Here's the drawing with two shaded views (mm, measured from the low corner). I have some questions. Coordinates: 2 decimals unless noted, no trailing zeros. Loops run counter-clockwise (first coordinate to the right, second up) from the corner with the lowest first, then second, coordinate; pieces in that order, holes last. Notation, with made-up numbers: (-37, 66) -> (-22, 66) arc R27 ccw to (-22, 93) -> close; hole circle Ø1 at (11, 86.5). An arc over 180 degrees is marked (long way). Answer as a JSON object with one key per item and string values. Group by question number.
1) I want a section at D-D (y = 41). Write out the boundary of the cut face in (x, z), then the cut area to 3 significant figures.
2) I want a section at A-A (y = 25.5). Write out the boundary of the cut face in (x, z) (3 decimals).
3) I want a section at C-C (x = 0.7). Write out the boundary of the cut face in (y, z), then the cut area to 4 significant figures.
4) I need wall thicknesses on probe 1 along Z at (x, y) = (0.8, 32.5); probe 2 along Y at (x, z) = (4.6, 14). Which ranges of each line are inside material? Lowest first, please. Write a range as [from, to].
5) I'm going to push flat-ended pins straight in: pin 1 (3 mm diameter, centred on x = 4, z = 25.5, fed in from -Y); pin 2 (8 mm diameter, centred on y = 29, z = 23.5, fed in from -X); pin 3 (2 mm diameter, centred on x = 1, y = 32.5, fed in from +Z); pin 4 (0.8 mm diameter, centred on x = 1, y = 25, fed in from -Z). Where does each tip first touch, or does it pass through?
6) I want a section at B-B (z = 26). Write out the boundary of the cut face in (x, y).
7) If we mould it in two halves opening along Z, with no side actions, what happens to the marked faces 1 and 2? For each: +Z half, -Z half, draft (parallel to the pull), parting line (faces both ways), or undercut.
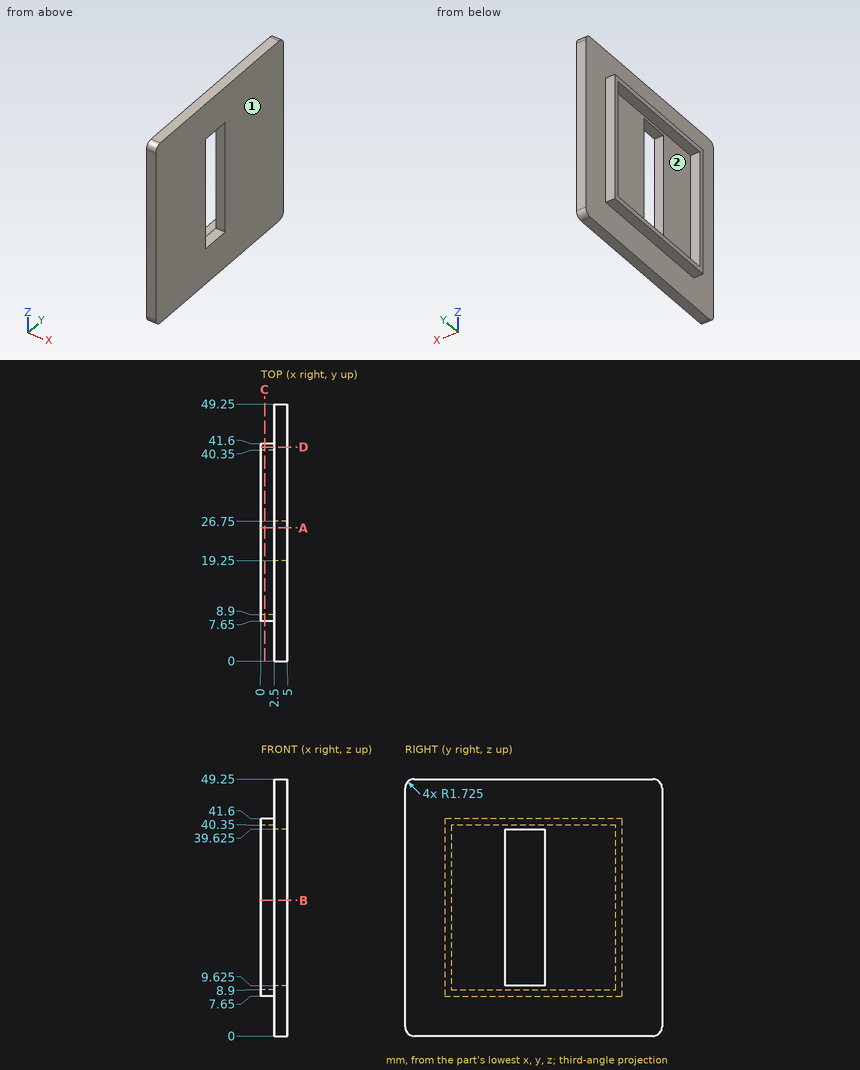
Determined:
{
 "1": {"outline": "(0, 7.65) -> (2.5, 7.65) -> (2.5, 0) -> (5, 0) -> (5, 49.25) -> (2.5, 49.25) -> (2.5, 41.6) -> (0, 41.6) -> close", "area": "208 mm^2"},
 "2": {"outline": "(0, 7.65) -> (2.5, 7.65) -> (2.5, 0) -> (5, 0) -> (5, 9.625) -> (2.5, 9.625) -> (2.5, 8.9) -> (0, 8.9) -> close; (0, 40.35) -> (2.5, 40.35) -> (2.5, 39.625) -> (5, 39.625) -> (5, 49.25) -> (2.5, 49.25) -> (2.5, 41.6) -> (0, 41.6) -> close"},
 "3": {"outline": "(7.65, 7.65) -> (41.6, 7.65) -> (41.6, 41.6) -> (7.65, 41.6) -> close; hole (8.9, 8.9) -> (40.35, 8.9) -> (40.35, 40.35) -> (8.9, 40.35) -> close", "area": "163.5 mm^2"},
 "4": {"probe 1": "[7.65, 8.9], [40.35, 41.6]", "probe 2": "[0, 19.25], [26.75, 49.25]"},
 "5": {"pin 1": "y = 0", "pin 2": "x = 2.5", "pin 3": "z = 41.6", "pin 4": "z = 7.65"},
 "6": {"outline": "(0, 7.65) -> (2.5, 7.65) -> (2.5, 0) -> (5, 0) -> (5, 19.25) -> (2.5, 19.25) -> (2.5, 8.9) -> (0, 8.9) -> close; (0, 40.35) -> (2.5, 40.35) -> (2.5, 26.75) -> (5, 26.75) -> (5, 49.25) -> (2.5, 49.25) -> (2.5, 41.6) -> (0, 41.6) -> close"},
 "7": {"face 1": "draft", "face 2": "undercut"}
}
